```python
from build123d import *

# Parameters (mm, degrees)
BOSS_EXTRUDE3_START = 1
BOSS_EXTRUDE3_DEPTH = 17
CUT_EXTRUDE1_START  = -1
CUT_EXTRUDE1_DEPTH  = 15


with BuildPart() as part:
    # Sketch1 → Boss-Extrude3 (new body)
    with BuildSketch(Plane.XY.offset(BOSS_EXTRUDE3_START)):
        with BuildLine():
            Line((22.4, 5.7), (22.4, 28.7))
            Line((22.4, 28.7), (27.4, 28.7))
            Line((27.4, 28.7), (55.753018587, 22.683636365))
            Line((55.753018587, 22.683636365), (60.914628912, 17.309586353))
            ThreePointArc((60.914628912, 17.309586353), (44.261162639, 13.072852444), (28.739278089, 5.7))
            Line((28.739278089, 5.7), (22.4, 5.7))
        make_face()
    extrude(amount=-BOSS_EXTRUDE3_DEPTH)

    # Sketch2 → Cut-Extrude1 (cut)
    with BuildSketch(Plane.XY.offset(1).offset(CUT_EXTRUDE1_START)):
        with BuildLine():
            Line((22.4, 6.7), (28.46302932, 6.7))
            ThreePointArc((28.46302932, 6.7), (43.722391124, 13.941290059), (60.06988402, 18.189098949))
            Line((60.06988402, 18.189098949), (56.469277883, 21.937897528))
            Line((56.469277883, 21.937897528), (54.449845351, 21.937897528))
            Line((54.449845351, 21.937897528), (27.295070739, 27.7))
            Line((27.295070739, 27.7), (22.4, 27.7))
            Line((22.4, 27.7), (22.4, 6.7))
        make_face()
    extrude(amount=-CUT_EXTRUDE1_DEPTH, mode=Mode.SUBTRACT)


solid = part.part
```
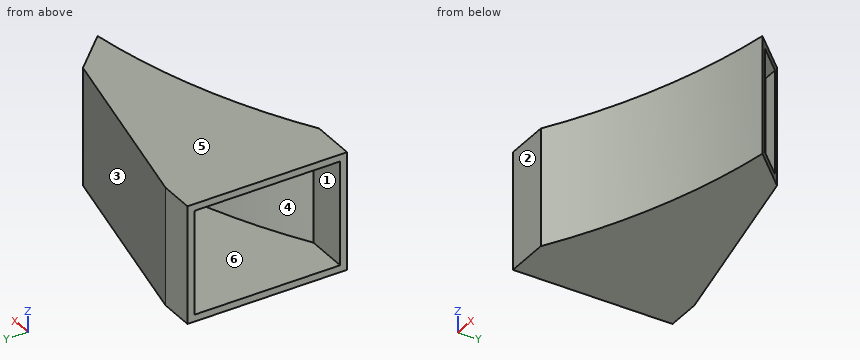
The model under review builds one solid part; all positions refer to its coordinate system, in mm. Face numbers are marked on the shaded views. A direction names the side the tool comes from. Round coordinates to 2 decimals unless told otherwise and drop trailing zeros. Loops run counter-clockwise (first coordinate to the right, second up) from the corner with the lowest first, then second, coordinate; pieces in that order, holes last. Notation, with made-up numbers: M 70,22.5 L 97,22.5 A19 cw 97,40.5 Z; hole C 34,64 d4. An arc over 180 degrees is marked long. Write item = value, one per line.
Item 1: Take a section at B-B on z = -2.75. Write out the cut boundary in (x, y), then the cut area to 3 significant figures.
Return value:
outline = M 22.4,5.7 L 28.74,5.7 A88.57 cw 60.91,17.31 L 60.07,18.19 A89.57 ccw 28.46,6.7 L 22.4,6.7 Z; M 22.4,27.7 L 27.3,27.7 L 54.45,21.94 L 56.47,21.94 L 55.75,22.68 L 27.4,28.7 L 22.4,28.7 Z
area = 74.4 mm2
Item 2: Machinability: for the marked faces 1 and 2, which of the approach directions +Z, -Z, +X, -X, +Y, -Y give a long, thin tool a straight path to every point of the face, cutting with its end or side? Answer none if there is none.
Return value:
face_1 = -X
face_2 = +Z, -Z, +X, -X, -Y
Item 3: Take a section at A-A on x = 25.5. Write out the cut boundary in (y, z).
Return value:
outline = M 5.7,-16 L 28.7,-16 L 28.7,1 L 5.7,1 Z; hole M 6.7,-15 L 27.7,-15 L 27.7,0 L 6.7,0 Z
Item 4: Take a section at D-D on y = 24. Write out the cut boundary in (x, z), then the cut area to 3 significant figures.
Return value:
outline = M 22.4,-16 L 49.55,-16 L 49.55,1 L 22.4,1 L 22.4,0 L 44.73,0 L 44.73,-15 L 22.4,-15 Z
area = 127 mm2
Item 5: The part is to be moulded in two halves that separate along Z. For the marked faces 3, 4, 5 and 6, say which applies: released by +Z, released by -Z, zero draft, split by the parting line, or undercut.
Return value:
face_3 = zero draft
face_4 = undercut
face_5 = released by +Z
face_6 = undercut
Item 6: For line 1 (Z direction, x = 31.5, y = 17); line 2 (Y direction, x = 25, z = -6.75); line 3 (Y direction, x = 49, z = -1), list the stretches that pass through material, from the lowest coordinate up. Write a range as [from, to].
Return value:
line_1 = [-16, -15], [0, 1]
line_2 = [5.7, 6.7], [27.7, 28.7]
line_3 = [14.63, 15.68], [23.09, 24.12]
Item 7: Take a section at C-C on y = 19. Write out the cut boundary in (x, z), then the cut area to 3 significant figures.
Return value:
outline = M 22.4,-16 L 59.29,-16 L 59.29,-15 L 22.4,-15 Z; M 22.4,0 L 59.29,0 L 59.29,1 L 22.4,1 Z
area = 73.8 mm2
Item 8: Insertion check: P1, Ø8, axis at x = 41, z = -6, coming from the +Y side; P2, Ø2, axis at x = 52.5, y = 13, coming from the -Z side; P3, Ø1, axis at x = 55.5, z = -6, coming from the -Y side; P4, Ø8, axis at x = 35, z = -4.5, coming from the -Y side. Each pin has a flat end and moves straight along its axis. Give the tip position at first contact, or say it passes through.
Return value:
P1 = 26.66
P2 = through
P3 = 16.2
P4 = 7.01
